```python
from build123d import *

# Parameters (mm, degrees)
SKETCH1_W           = 40
SKETCH1_H           = 20
BOSS_EXTRUDE1_DEPTH = 28.7
SKETCH2_W           = 54.5
SKETCH2_H           = 20
BOSS_EXTRUDE2_DEPTH = 2.5
SKETCH3_W           = 40
SKETCH3_H           = 20
BOSS_EXTRUDE3_DEPTH = 5.8
SKETCH4_R           = 6
BOSS_EXTRUDE4_DEPTH = 7.1
SKETCH5_R           = 2.55
CUT_EXTRUDE3_DEPTH  = 7.1


with BuildPart() as part:
    # Sketch1 → Boss-Extrude1 (new body)
    with BuildSketch(Plane(origin=(0, 0, 0), x_dir=(1, 0, 0), z_dir=(0, 1, 0))):
        Rectangle(SKETCH1_W, SKETCH1_H)
    extrude(amount=BOSS_EXTRUDE1_DEPTH)

    # Sketch2 → Boss-Extrude2 (add)
    with BuildSketch(Plane(origin=(0, 28.7, 0), x_dir=(1, 0, 0), z_dir=(0, 1, 0))):
        Rectangle(SKETCH2_W, SKETCH2_H)
    extrude(amount=BOSS_EXTRUDE2_DEPTH)

    # Sketch3 → Boss-Extrude3 (add)
    with BuildSketch(Plane(origin=(0, 31.2, 0), x_dir=(1, 0, 0), z_dir=(0, 1, 0))):
        Rectangle(SKETCH3_W, SKETCH3_H)
    extrude(amount=BOSS_EXTRUDE3_DEPTH)

    # Sketch4 → Boss-Extrude4 (add)
    with BuildSketch(Plane(origin=(0, 37, 0), x_dir=(1, 0, 0), z_dir=(0, 1, 0))):
        with Locations((9.9, 0)):
            Circle(SKETCH4_R)
    extrude(amount=BOSS_EXTRUDE4_DEPTH)

    # Sketch5 → Cut-Extrude3 (cut)
    with BuildSketch(Plane(origin=(0, 31.2, 0), x_dir=(1, 0, 0), z_dir=(0, 1, 0))):
        with Locations((-24.75, 5)):
            Circle(SKETCH5_R)
        with Locations((-24.75, -5)):
            Circle(SKETCH5_R)
        with Locations((24.75, -5)):
            Circle(SKETCH5_R)
        with Locations((24.75, 5)):
            Circle(SKETCH5_R)
    extrude(amount=-CUT_EXTRUDE3_DEPTH, mode=Mode.SUBTRACT)


solid = part.part
```
Design review of the part built by this model. Coordinates are the model's own, in mm. A direction names the side the tool comes from. Give positions to 0.01 mm unless a question says otherwise; leave off trailing zeros. Order: outer loops, then holes, each group sorted by start corner. A loop starts at its lowest first (then second) coordinate and runs counter-clockwise, first axis right, second up. Notation, with made-up numbers: (89, -4.5) -> (132, -4.5) arc R15 cw to (132, 18.5) -> close; hole circle Ø6 at (87.5, 7.25). An arc over 180 degrees is marked (long way). Write item = value, one per line. Start each with the question number.
(1) Mouldability with a two-part tool opening along X and no side actions: class faces 1 (the face through (-27.25, 30, 0)), 2 (the face through (20, 14, 0)), 3 (the face through (-22.2, 30, -4.9)) as +X half, -X half, draft (parallel to the pull), parting line (faces both ways), or undercut.
(2) To check wall thickness, follow line 1 along Z through (x, y) = (24.75, 29.4); line 2 along Z through (x, y) = (24, 30); line 3 along X through (y, z) = (29.3, 5). State the ranges of each line that lie inside material, in increasing order.
(3) For faces 4 (the face through (-24, 31.2, 0)), 5 (the face through (-24, 28.7, 0)), 6 (the face through (20, 34, 0)), 7 (the face through (24, 28.7, 0)), list the 3-axis set-ups (+Z, -Z, +X, -X, +Y, -Y) from which the entire face can be reached by the end or side of a thin tool; tool diameter is ignored.
(4) We need section A-A on x = 24.75. Write out the cut boundary in (y, z), plus the area to 3 significant figures.
(5) For pin 1 (1 mm diameter, centred on y = 9.5, z = 7, fed in from -X); pin 2 (4 mm diameter, centred on x = 24.75, z = 5, fed in from -Y); pin 3 (6 mm diameter, centred on x = 24.75, z = -5, fed in from +Y); pin 4 (10 mm diameter, centred on y = 11, z = -0.5, fed in from +X), all flat-tipped, find the tip position at first contact; note any pin that passes through.
(6) We need section D-D on y = 12. Write out the cut boundary in (x, z), plus the area to 3 significant figures.
(7) We need section B-B on z = 0. Write out the cut boundary in (x, y).
(8) We need section C-C on x = 9.9. Write out the cut boundary in (y, z).
Numbers:
q1.face_1 = -X half
q1.face_2 = +X half
q1.face_3 = undercut
q2.line_1 = -10 to -7.55, -2.45 to 2.45, 7.55 to 10
q2.line_2 = -10 to -7.44, -2.56 to 2.56, 7.44 to 10
q2.line_3 = -22.2 to 22.2
q3.face_4 = +Z, -Z, -X, +Y
q3.face_5 = +Z, -Z, -X, -Y
q3.face_6 = +Z, -Z, +X, +Y
q3.face_7 = +Z, -Z, +X, -Y
q4.outline = (28.7, -10) -> (31.2, -10) -> (31.2, -7.55) -> (28.7, -7.55) -> close; (28.7, -2.45) -> (31.2, -2.45) -> (31.2, 2.45) -> (28.7, 2.45) -> close; (28.7, 7.55) -> (31.2, 7.55) -> (31.2, 10) -> (28.7, 10) -> close
q4.area = 24.5 mm^2
q5.pin_1 = -20
q5.pin_2 = through
q5.pin_3 = 31.2
q5.pin_4 = 20
q6.outline = (-20, -10) -> (20, -10) -> (20, 10) -> (-20, 10) -> close
q6.area = 800 mm^2
q7.outline = (-27.25, 28.7) -> (-20, 28.7) -> (-20, 0) -> (20, 0) -> (20, 28.7) -> (27.25, 28.7) -> (27.25, 31.2) -> (20, 31.2) -> (20, 37) -> (15.9, 37) -> (15.9, 44.1) -> (3.9, 44.1) -> (3.9, 37) -> (-20, 37) -> (-20, 31.2) -> (-27.25, 31.2) -> close
q8.outline = (0, -10) -> (37, -10) -> (37, -6) -> (44.1, -6) -> (44.1, 6) -> (37, 6) -> (37, 10) -> (0, 10) -> close
